Job drawing, mm, ordinate dimensions from the low corner. One solid piece. Give positions to 0.01 mm unless a question says otherwise; leave off trailing zeros. Write each loop counter-clockwise with the first axis right and the second up, starting at its lowest first coordinate (ties: lowest second). Pieces come first, ordered by that corner, then holes. Notation, with made-up numbers: (48.25, 13.5) -> (66.25, 13.5) arc R4 ccw to (66.25, 19.5) -> close; hole circle Ø6 at (70.25, -5.5). An arc over 180 degrees is marked (long way). Put each result on its own line as item: value. Start each with the question number.
Item 1: Two-plate mould, pull along Y, no slides. Class the marked faces 1, 2 and 3: pulls with the +Y half, pulls with the -Y half, needs draft (parallel to the pull), parting line crosses it, or undercut.
Item 2: Flat gauge pins, fed straight in: pin 1 Ø1.5 at (x, z) = (8.5, 8.5) entering from +Y; pin 2 Ø1.5 at (x, y) = (9.5, 6.5) entering from -Z; pin 3 Ø5 at (y, z) = (4, 7) entering from -X; pin 4 Ø5 at (x, z) = (5.5, 1.5) entering from -Y. Where does each tip first touch, or does it go through?
Item 3: Slice it at A-A, the plane z = 5.5. List the corners of the cut face in (x, y).
Item 4: Slice it at B-B, the plane x = 8.5. List the corners of the cut face in (y, z).
Item 5: Slice it at D-D, the plane z = 4.25. List the corners of the cut face in (x, y), plus the area to 3 significant figures.
Item 6: Drill centre lines: line 1 along X through (y, z) = (2.75, 8); line 2 along Y through (x, z) = (9.5, 5); line 3 along Z through (x, y) = (7.75, 7). Where is each one in solid material? Low to high.
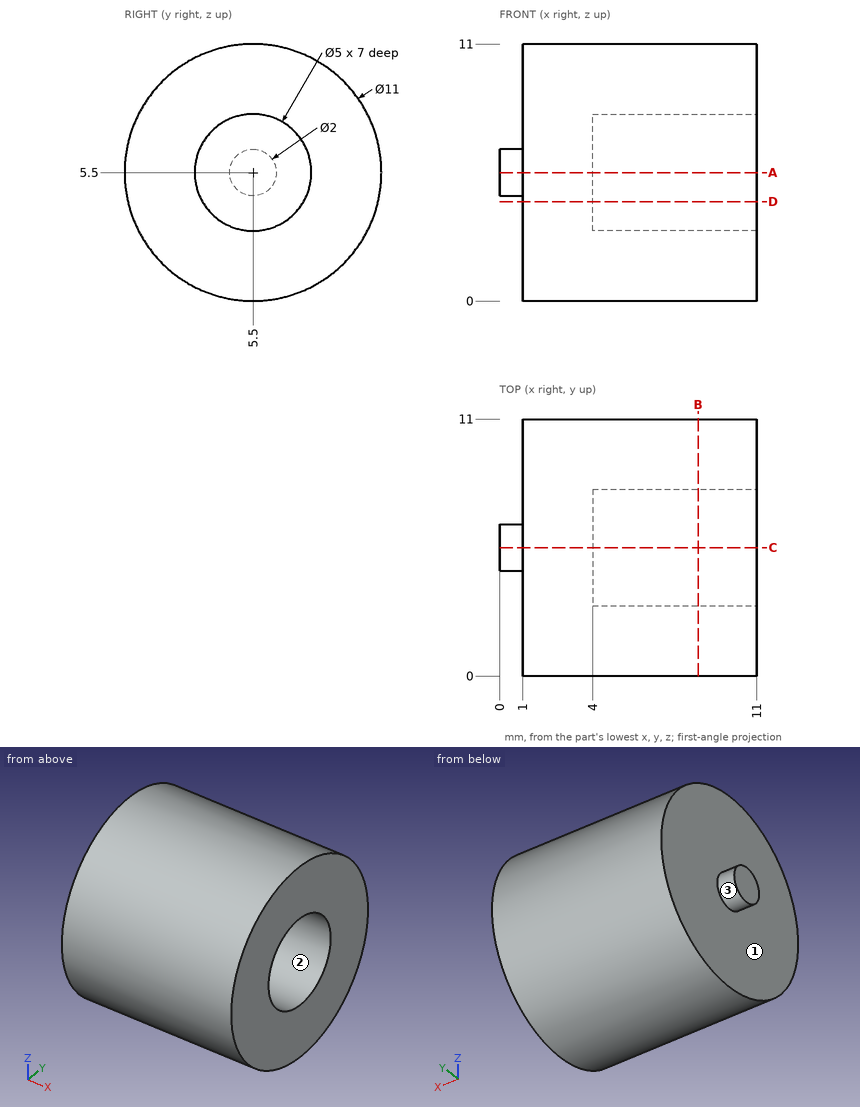
Values follow:
1. face 1: needs draft
1. face 2: undercut
1. face 3: parting line crosses it
2. pin 1: y = 10.52
2. pin 2: z = 0.01
2. pin 3: x = 0
2. pin 4: y = 0.21
3. outline: (0, 4.5) -> (1, 4.5) -> (1, 0) -> (11, 0) -> (11, 3) -> (4, 3) -> (4, 8) -> (11, 8) -> (11, 11) -> (1, 11) -> (1, 6.5) -> (0, 6.5) -> close
4. outline: circle Ø11 at (5.5, 5.5); hole circle Ø5 at (5.5, 5.5)
5. outline: (1, 0.14) -> (11, 0.14) -> (11, 3.33) -> (4, 3.33) -> (4, 7.67) -> (11, 7.67) -> (11, 10.86) -> (1, 10.86) -> close
5. area: 76.8 mm2
6. line 1: 1 to 11
6. line 2: 0.02 to 3.05, 7.95 to 10.98
6. line 3: 0.21 to 3.5, 7.5 to 10.79
